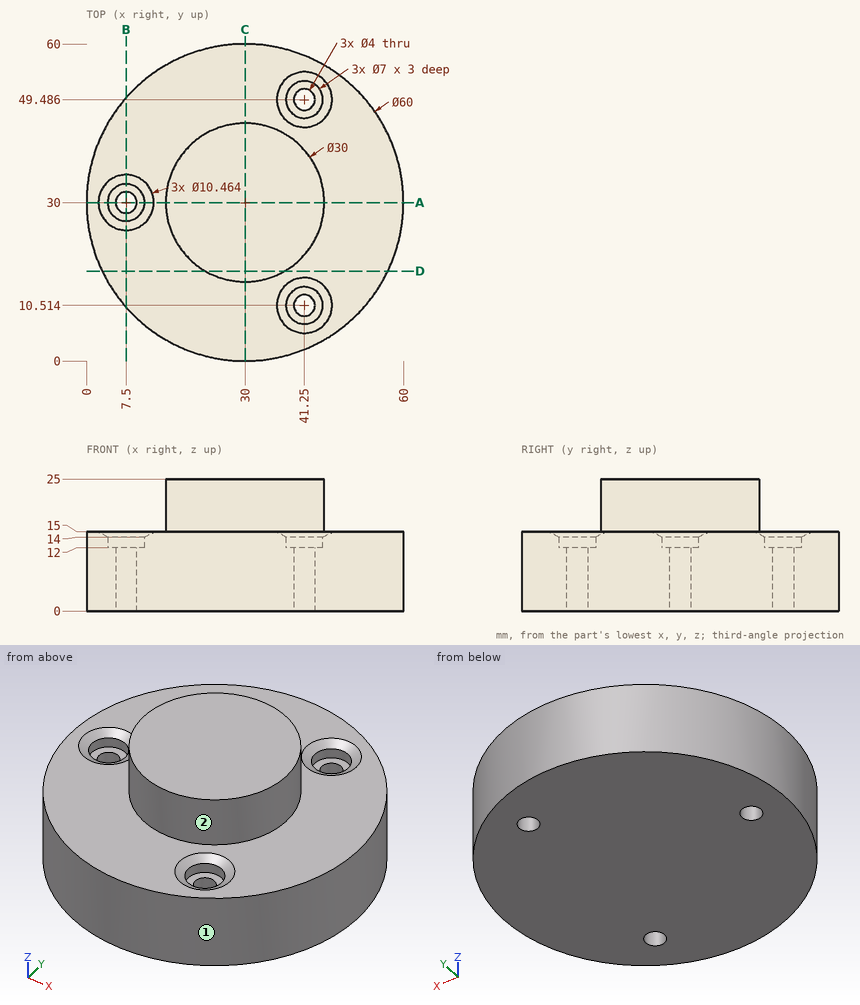
Job drawing, mm, ordinate dimensions from the low corner. One solid piece. A direction names the side the tool comes from. Give positions to 0.01 mm unless a question says otherwise; leave off trailing zeros. Order: outer loops, then holes, each group sorted by start corner. A loop starts at its lowest first (then second) coordinate and runs counter-clockwise, first axis right, second up. Notation, with made-up numbers: (34.5, 80) -> (41.5, 80) arc R25 cw to (41.5, 95) -> close; hole circle Ø10 at (-37.75, -5). An arc over 180 degrees is marked (long way). Return JSON: item names as keys, results as strings.
Q1. Which spindle directions (+Z, -Z, +X, -X, +Y, -Y) get a long thin tool onto all of the face, cutting with end or side? Do the marked faces 1 and 2. Say none if no direction does.
Working result:
{"face 1": "+Z, -Z", "face 2": "+Z"}
Q2. Saw through at B-B (x = 7.5). Write the cut outline in (y, z).
Working result:
{"outline": "(10.16, 0) -> (28, 0) -> (28, 12) -> (26.5, 12) -> (26.5, 14) -> (24.77, 15) -> (10.16, 15) -> close; (32, 0) -> (49.84, 0) -> (49.84, 15) -> (35.23, 15) -> (33.5, 14) -> (33.5, 12) -> (32, 12) -> close"}
Q3. Drill centre lines: line 1 (Y direction, x = 41.25, z = 6.25) (1 decimal); line 2 (Z direction, x = 49, y = 26); line 3 (Z direction, x = 5, y = 28). Where is each one in solid material? Low to high.
Working result:
{"line 1": "2.2 to 8.5, 12.5 to 47.5, 51.5 to 57.8", "line 2": "0 to 15", "line 3": "0 to 12"}
Q4. Flat gauge pins, fed straight in: pin 1 (4 mm diameter, centred on x = 8, z = 16.5, fed in from -Y) (1 decimal); pin 2 (6.5 mm diameter, centred on x = 41.25, y = 10.51, fed in from +Z); pin 3 (6 mm diameter, centred on x = 36.5, z = 9.5, fed in from -Y) (1 decimal). Where does each tip first touch, or does it go through?
Working result:
{"pin 1": "y = 8.3", "pin 2": "z = 12", "pin 3": "y = 0.2"}
Q5. Saw through at A-A (y = 30). Write the cut outline in (x, z).
Working result:
{"outline": "(0, 0) -> (5.5, 0) -> (5.5, 12) -> (4, 12) -> (4, 14) -> (2.27, 15) -> (0, 15) -> close; (9.5, 0) -> (60, 0) -> (60, 15) -> (45, 15) -> (45, 25) -> (15, 25) -> (15, 15) -> (12.73, 15) -> (11, 14) -> (11, 12) -> (9.5, 12) -> close"}
Q6. Saw through at C-C (x = 30). Write the cut outline in (y, z).
Working result:
{"outline": "(0, 0) -> (60, 0) -> (60, 15) -> (45, 15) -> (45, 25) -> (15, 25) -> (15, 15) -> (0, 15) -> close"}
Q7. Saw through at D-D (y = 17). Write the cut outline in (x, z), then the cut area to 3 significant figures.
Working result:
{"outline": "(2.96, 0) -> (57.04, 0) -> (57.04, 15) -> (37.48, 15) -> (37.48, 25) -> (22.52, 25) -> (22.52, 15) -> (2.96, 15) -> close", "area": "961 mm²"}
